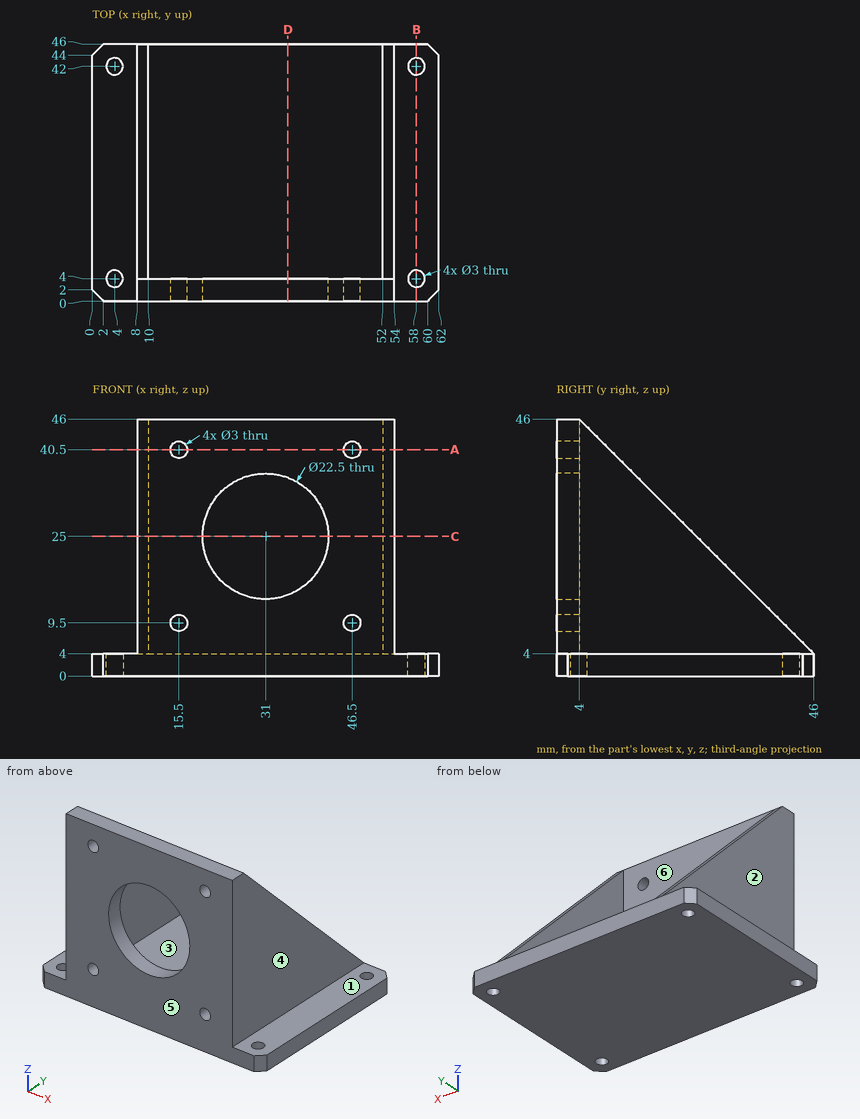
The figure shows three views and two pictorial views of one solid part (mm, origin at its lowest corner). Answer the questions. A direction names the side the tool comes from. Coordinates: 2 decimals unless noted, no trailing zeros. Loops run counter-clockwise (first coordinate to the right, second up) from the corner with the lowest first, then second, coordinate; pieces in that order, holes last. Notation, with made-up numbers: (6.5, 31.25) -> (22.5, 31.25) arc R19 cw to (22.5, 38.25) -> close; hole circle Ø7 at (71, -12). An arc over 180 degrees is marked (long way). Write item = value, one per line. Start each with the question number.
1) A cutting plane is placed at C-C (z = 25). Give the vertices of the cut face in (x, y), then the cut area to 3 significant figures.
2) A cutting plane is placed at B-B (x = 58). Give the vertices of the cut face in (y, z).
3) Given pin 1 Ø12 at (x, y) = (10, 38) entering from +Z; pin 2 Ø2.5 at (x, y) = (56.5, 22.5) entering from +Z; pin 3 Ø4 at (x, z) = (46.5, 40.5) entering from +Y, each flat-ended and moving along its own axis, determine where each tip first touches the part or whether it passes through.
4) A cutting plane is placed at D-D (x = 35). Give the vertices of the cut face in (y, z), then the cut area to 3 significant figures.
5) Straight lines are drawn through the part: line 1 (Y direction, x = 4, z = 1); line 2 (X direction, y = 25, z = 20.5); line 3 (Z direction, x = 15, y = 24). For each, find the intervals that lie inside material, in ascending order. Write a range as from..to.
6) The mould has two halves that part along X. Classify the marked faces 1, 2 and 3: released by +X, released by -X, zero draft, split by the parting line, or undercut.
7) A tool of negligible diameter and unlimited length cuts with its end or side. For the marked faces 4, 5 and 6, from which of +Z, -Z, +X, -X, +Y, -Y can it reach the whole face along a straight path? Write none if from no direction.
8) A cutting plane is placed at A-A (z = 40.5). Give the vertices of the cut face in (x, y), then the cut area to 3 significant figures.
Responses:
q1.outline = (8, 0) -> (19.75, 0) -> (19.75, 4) -> (10, 4) -> (10, 25) -> (8, 25) -> close; (42.25, 0) -> (54, 0) -> (54, 25) -> (52, 25) -> (52, 4) -> (42.25, 4) -> close
q1.area = 178 mm²
q2.outline = (0, 0) -> (2.5, 0) -> (2.5, 4) -> (0, 4) -> close; (5.5, 0) -> (40.5, 0) -> (40.5, 4) -> (5.5, 4) -> close; (43.5, 0) -> (46, 0) -> (46, 4) -> (43.5, 4) -> close
q3.pin_1 = 18
q3.pin_2 = 4
q3.pin_3 = 4
q4.outline = (0, 0) -> (46, 0) -> (46, 4) -> (4, 4) -> (4, 14.49) -> (0, 14.49) -> close; (0, 35.51) -> (4, 35.51) -> (4, 46) -> (0, 46) -> close
q4.area = 268 mm²
q5.line_1 = 0..2.5, 5.5..40.5, 43.5..46
q5.line_2 = 8..10, 52..54
q5.line_3 = 0..4
q6.face_1 = zero draft
q6.face_2 = released by -X
q6.face_3 = undercut
q7.face_4 = +Z, +X, +Y, -Y
q7.face_5 = +Z, -Z, +X, -X, -Y
q7.face_6 = +Z, +Y
q8.outline = (8, 0) -> (14, 0) -> (14, 4) -> (10, 4) -> (10, 9.5) -> (8, 9.5) -> close; (17, 0) -> (45, 0) -> (45, 4) -> (17, 4) -> close; (48, 0) -> (54, 0) -> (54, 9.5) -> (52, 9.5) -> (52, 4) -> (48, 4) -> close
q8.area = 182 mm²
